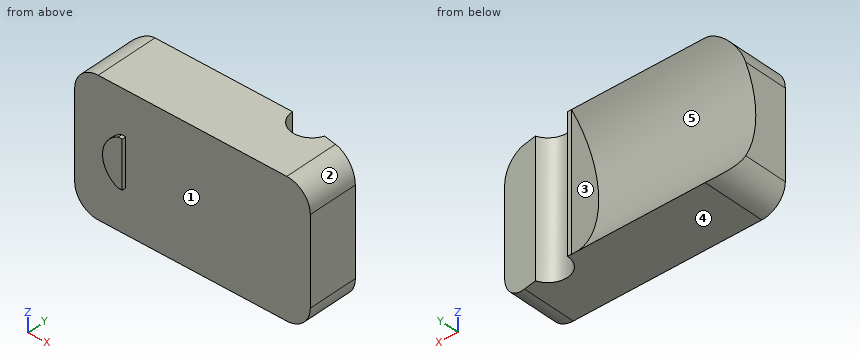
```python
from build123d import *

# Parameters (mm, degrees)
SKETCH1_W           = 60
SKETCH1_H           = 34
BOSS_EXTRUDE1_DEPTH = 16
SKETCH6_R           = 22.671568098
CUT_EXTRUDE4_DEPTH  = 40
SKETCH2_R           = 5
CUT_EXTRUDE1_DEPTH  = 71.795480082
FILLET1_R           = 6
CUT_EXTRUDE3_DEPTH  = 71.795480152
BOSS_EXTRUDE2_DEPTH = 1


with BuildPart() as part:
    # Sketch1 → Boss-Extrude1 (new body)
    with BuildSketch(Plane(origin=(0, 0, 0), x_dir=(1, 0, 0), z_dir=(0, 1, 0))):
        with Locations((30, 17)):
            Rectangle(SKETCH1_W, SKETCH1_H)
    extrude(amount=BOSS_EXTRUDE1_DEPTH)

    # Sketch6 → Cut-Extrude4 (cut)
    with BuildSketch(Plane.ZY):
        with Locations((-17, 31)):
            Circle(SKETCH6_R)
    extrude(amount=-CUT_EXTRUDE4_DEPTH, mode=Mode.SUBTRACT)

    # Sketch2 → Cut-Extrude1 (cut, through all)
    with BuildSketch(Plane.XY):
        with Locations((46, 16)):
            Circle(SKETCH2_R)
    extrude(amount=-CUT_EXTRUDE1_DEPTH, mode=Mode.SUBTRACT)

    # Fillet1
    fillet1_edges = [part.edges().sort_by_distance(p)[0] for p in [
        (0, 8, -34),
        (60, 8, -34),
        (60, 8, 0),
        (0, 8, 0),
    ]]
    fillet(fillet1_edges, radius=FILLET1_R)

    # Sketch5 → Cut-Extrude3 (cut, through all)
    with BuildSketch(Plane.XY):
        Polygon((50.705913613, 14.310509822), (60, 12.692705636), (60, 16), (51, 16), align=None)
    extrude(amount=-CUT_EXTRUDE3_DEPTH, mode=Mode.SUBTRACT)

    # Sketch7 → Boss-Extrude2 (add)
    with BuildSketch(Plane.XZ):
        with BuildLine():
            Line((13, -11), (13, -23))
            Line((13, -23), (12, -23))
            ThreePointArc((12, -23), (8, -17), (12, -11))
            Line((12, -11), (13, -11))
        make_face()
    extrude(amount=BOSS_EXTRUDE2_DEPTH)


solid = part.part
```
Check sheet for the modelled part. Datum: model origin and axes. Units: mm. Face numbers are marked on the shaded views. A direction names the side the tool comes from. Give positions to 0.01 mm unless a question says otherwise; leave off trailing zeros. Order: outer loops, then holes, each group sorted by start corner. A loop starts at its lowest first (then second) coordinate and runs counter-clockwise, first axis right, second up. Notation, with made-up numbers: M -19,10 L 2,10 A29 cw 2,47 Z; hole C 3.25,-4 d2. An arc over 180 degrees is marked long. Answer in a Markdown table with one row per item.
1) Access from +Z, -Z, +X, -X, +Y, -Y to the whole of each face (thin tool, end or side, straight path). Record for the marked faces 4 and 5.
Filled sheet:
| item | result |
|---|---|
| face 4 | -Z, +X, -X, +Y, -Y |
| face 5 | -X, +Y |
2) Cross-section at A-A, the plane y = 12. Enter the section's corners in (x, z), plus the area to 3 significant figures.
Filled sheet:
| item | result |
|---|---|
| outline | M 0.16,-29.37 A6 ccw 6,-34 L 43,-34 L 43,0 L 6,0 A6 ccw 0.16,-4.63 L 40,-4.63 L 40,-29.37 Z; M 49,-34 L 54,-34 A6 ccw 60,-28 L 60,-6 A6 ccw 54,0 L 49,0 Z |
| area | 816 mm2 |
3) Cross-section at B-B, the plane z = -19.5. Enter the section's corners in (x, y).
Filled sheet:
| item | result |
|---|---|
| outline | M 0,0 L 8.5,0 L 8.5,-1 L 13,-1 L 13,0 L 60,0 L 60,12.69 L 50.71,14.31 A5 cw 41,16 L 40,16 L 40,8.47 L 0,8.47 Z |
4) Release check for a two-part mould opening along Z. For the marked faces 1, 2 and 3 record: +Z half, -Z half, draft (parallel to the pull), parting line (faces both ways), or undercut.
Filled sheet:
| item | result |
|---|---|
| face 1 | draft |
| face 2 | +Z half |
| face 3 | undercut |
5) Gauge pin test, flat ends, axial feed: P1, Ø0.8, axis at x = 12.5, y = -0.5, coming from the -Z side; P2, Ø1, axis at x = 30.5, z = -22, coming from the -Y side; P3, Ø0.5, axis at y = -0.5, z = -19, coming from the +X side. Record the tip position at first contact, or that the pin passes through.
Filled sheet:
| item | result |
|---|---|
| P1 | stops at z = -23 |
| P2 | stops at y = 0 |
| P3 | stops at x = 13 |
6) Cross-section at D-D, the plane x = 17. Enter the section's corners in (y, z).
Filled sheet:
| item | result |
|---|---|
| outline | M 0,-34 L 16,-34 A22.67 cw 16,0 L 0,0 Z |
7) Thickness scan on L1, parallel to X at y = 12.5, z = -12; L2, parallel to Z at x = 20.5, y = 13.5; L3, parallel to Z at x = 10.5, y = 15.25. Record the ranges inside material, lowest first. Write a range as [from, to].
Filled sheet:
| item | result |
|---|---|
| L1 | x = [40, 42.43], [49.57, 60] |
| L2 | z = [-34, -31.41], [-2.59, 0] |
| L3 | z = [-34, -33.31], [-0.69, 0] |
8) Cross-section at C-C, the plane y = 4.5. Enter the section's corners in (x, z).
Filled sheet:
| item | result |
|---|---|
| outline | M 0,-28 A6 ccw 6,-34 L 54,-34 A6 ccw 60,-28 L 60,-6 A6 ccw 54,0 L 6,0 A6 ccw 0,-6 Z |
